from build123d import *

# Parameters (mm, degrees)
DODANIE_WYCI_GNI_CIE1_DEPTH = 5
SZKIC1_R                    = 3.5
WYTNIJ_WYCI_GNI_CIE1_DEPTH  = 88.4
SZKIC3_R                    = 1.5
WYTNIJ_WYCI_GNI_CIE3_DEPTH  = 5
SZKIC5_R                    = 3
WYTNIJ_WYCI_GNI_CIE4_DEPTH  = 2.4
DODANIE_WYCI_GNI_CIE2_START = 5
DODANIE_WYCI_GNI_CIE2_DEPTH = 5
SZKIC7_R                    = 3.5
WYTNIJ_WYCI_GNI_CIE5_DEPTH  = 5
SZKIC8_R                    = 3.5
WYTNIJ_WYCI_GNI_CIE6_DEPTH  = 5
SZKIC9_R                    = 1.5
WYTNIJ_WYCI_GNI_CIE7_DEPTH  = 3
SZKIC10_R                   = 2.85
WYTNIJ_WYCI_GNI_CIE8_DEPTH  = 2
SZKIC11_W                   = 7
SZKIC11_H                   = 5
WYTNIJ_WYCI_GNI_CIE9_DEPTH  = 3.5


with BuildPart() as part:
    # outer-wire → Dodanie-wyciągnięcie1 (new body)
    with BuildSketch(Plane.XY):
        with BuildLine():
            Line((-24, -24.53020641), (62.5, -24.53020641))
            ThreePointArc((62.5, -24.53020641), (65.803504247, -23.968789974), (68.736080178, -22.347578348))
            Line((68.736080178, -22.347578348), (89, -6.182628062))
            ThreePointArc((89, -6.182628062), (91.932575931, -4.561416436), (95.236080178, -4))
            Line((95.236080178, -4), (167, -4))
            ThreePointArc((167, -4), (172.310885546, -5.526836794), (176, -9.641101056))
            Line((176, -9.641101056), (192, -39.280484771))
            ThreePointArc((192, -39.280484771), (195.676368139, -43.118069462), (200.799707694, -44.53020641))
            Line((200.799707694, -44.53020641), (271, -44.53020641))
            ThreePointArc((271, -44.53020641), (292.697243682, -34.454979346), (299, -11.3778078))
            Line((299, -11.3778078), (299, 70.236479581))
            ThreePointArc((299, 70.236479581), (290.082226047, 86.530998263), (273, 93.827270232))
            Line((273, 93.827270232), (-19, 110))
            ThreePointArc((-19, 110), (-33.142135624, 104.142135624), (-39, 90))
            Line((-39, 90), (-39, -9.53020641))
            ThreePointArc((-39, -9.53020641), (-34.606601718, -20.136808128), (-24, -24.53020641))
        make_face()
    extrude(amount=DODANIE_WYCI_GNI_CIE1_DEPTH)

    # Szkic1 → Wytnij-wyciągnięcie1 (cut)
    with BuildSketch(Plane(origin=(0, -24.53020641, 0), x_dir=(-1, 0, 0), z_dir=(0, -1, 0))):
        with Locations((19, 0)):
            Circle(SZKIC1_R)
    extrude(amount=-WYTNIJ_WYCI_GNI_CIE1_DEPTH, mode=Mode.SUBTRACT)

    # Szkic3 → Wytnij-wyciągnięcie3 (cut)
    with BuildSketch(Plane.XY.offset(5)):
        with Locations((-5, 77.5)):
            Circle(SZKIC3_R)
        with Locations((-29, 77.5)):
            Circle(SZKIC3_R)
        with Locations((-29, -12.5)):
            Circle(SZKIC3_R)
        with Locations((-29, 32.5)):
            Circle(SZKIC3_R)
        with Locations((-5, 32.5)):
            Circle(SZKIC3_R)
        with Locations((-5, -12.5)):
            Circle(SZKIC3_R)
    extrude(amount=-WYTNIJ_WYCI_GNI_CIE3_DEPTH, mode=Mode.SUBTRACT)

    # Szkic5 → Wytnij-wyciągnięcie4 (cut)
    with BuildSketch(Plane.XY.offset(5)):
        with Locations((-29, -12.5)):
            Circle(SZKIC5_R)
        with Locations((-29, 32.5)):
            Circle(SZKIC5_R)
        with Locations((-29, 77.5)):
            Circle(SZKIC5_R)
        with Locations((-5, 77.5)):
            Circle(SZKIC5_R)
        with Locations((-5, 32.5)):
            Circle(SZKIC5_R)
        with Locations((-5, -12.5)):
            Circle(SZKIC5_R)
    extrude(amount=-WYTNIJ_WYCI_GNI_CIE4_DEPTH, mode=Mode.SUBTRACT)

    # Szkic6 → Dodanie-wyciągnięcie2 (add)
    with BuildSketch(Plane(origin=(0, 0, 0), x_dir=(-1, 0, 0), z_dir=(0, 0, -1)).offset(DODANIE_WYCI_GNI_CIE2_START)):
        with BuildLine():
            Line((-8, -24.53020641), (-8, 108.504576357))
            Line((-8, 108.504576357), (-273, 93.827270232))
            ThreePointArc((-273, 93.827270232), (-290.082226047, 86.530998263), (-299, 70.236479581))
            Line((-299, 70.236479581), (-299, -11.3778078))
            ThreePointArc((-299, -11.3778078), (-292.697243682, -34.454979346), (-271, -44.53020641))
            Line((-271, -44.53020641), (-200.799707694, -44.53020641))
            ThreePointArc((-200.799707694, -44.53020641), (-195.676368139, -43.118069462), (-192, -39.280484771))
            Line((-192, -39.280484771), (-176, -9.641101056))
            ThreePointArc((-176, -9.641101056), (-172.310885546, -5.526836794), (-167, -4))
            Line((-167, -4), (-95.236080178, -4))
            ThreePointArc((-95.236080178, -4), (-91.932575931, -4.561416436), (-89, -6.182628062))
            Line((-89, -6.182628062), (-68.736080178, -22.347578348))
            ThreePointArc((-68.736080178, -22.347578348), (-65.803504247, -23.968789974), (-62.5, -24.53020641))
            Line((-62.5, -24.53020641), (-8, -24.53020641))
        make_face()
    extrude(amount=-DODANIE_WYCI_GNI_CIE2_DEPTH)

    # Szkic7 → Wytnij-wyciągnięcie5 (cut)
    with BuildSketch(Plane(origin=(0, 65.36979359, 0), x_dir=(-1, 0, 0), z_dir=(0, -1, 0))):
        with Locations((19, 0)):
            Circle(SZKIC7_R)
    extrude(amount=-WYTNIJ_WYCI_GNI_CIE5_DEPTH, mode=Mode.SUBTRACT)

    # Szkic8 → Wytnij-wyciągnięcie6 (cut)
    with BuildSketch(Plane(origin=(0, 73.36979359, 0), x_dir=(-1, 0, 0), z_dir=(0, -1, 0))):
        with Locations((19, 0)):
            Circle(SZKIC8_R)
    extrude(amount=-WYTNIJ_WYCI_GNI_CIE6_DEPTH, mode=Mode.SUBTRACT)

    # Szkic9 → Wytnij-wyciągnięcie7 (cut)
    with BuildSketch(Plane(origin=(0, 73.36979359, 0), x_dir=(-1, 0, 0), z_dir=(0, -1, 0))):
        with Locations((19, 0)):
            Circle(SZKIC9_R)
    extrude(amount=WYTNIJ_WYCI_GNI_CIE7_DEPTH, mode=Mode.SUBTRACT)

    # Szkic10 → Wytnij-wyciągnięcie8 (cut)
    with BuildSketch(Plane(origin=(0, 65.36979359, 0), x_dir=(-1, 0, 0), z_dir=(0, -1, 0))):
        with Locations((19, 0)):
            Circle(SZKIC10_R)
    extrude(amount=WYTNIJ_WYCI_GNI_CIE8_DEPTH, mode=Mode.SUBTRACT)

    # Szkic11 → Wytnij-wyciągnięcie9 (cut)
    with BuildSketch(Plane(origin=(0, 0, 0), x_dir=(-1, 0, 0), z_dir=(0, 0, -1))):
        with Locations((19, 75.86979359)):
            Rectangle(SZKIC11_W, SZKIC11_H)
        with Locations((19, 67.86979359)):
            Rectangle(SZKIC11_W, SZKIC11_H)
    extrude(amount=-WYTNIJ_WYCI_GNI_CIE9_DEPTH, mode=Mode.SUBTRACT)


solid = part.part
Work out the finished part from the listing and answer in its coordinate system (mm). A direction names the side the tool comes from. Give positions to 0.01 mm unless a question says otherwise; leave off trailing zeros. Loops run counter-clockwise (first coordinate to the right, second up) from the corner with the lowest first, then second, coordinate; pieces in that order, holes last. Notation, with made-up numbers: (-11, -24.5) - (47, -24.5) arc R27 cw to (47, 1.5) - close; hole circle Ø10 at (-22, 20). An arc over 180 degrees is marked (long way). Answer in a Markdown table with one row per item. Add a question column.
Q1. The part is cut by section C-C (x = 120). Determine the outline of the cut face in (y, z), and give its area (3 significant figures).
Q2. Each of these flat-tipped pins is pushed along its axis until it touches: P1, Ø5.5, axis at x = -29, y = 32.5, coming from the +Z side; P2, Ø8, axis at x = -29, y = -12.5, coming from the -Z side; P3, Ø1.5, axis at x = 205.5, z = 0.5, coming from the +Y side. Where does it stop, or does it pass through?
Q3. Determine the mould class of faces 1 (the flat face through (156, 33, -5)), 2 (the flat face through (-4, -11, 2.6)), 3 (the flat face through (29, -24.53, 0)) for opening direction Y: released by +Y, released by -Y, zero draft, split by the parting line, or undercut.
Q4. A tool of negligible diameter and unlimited length cuts with its end or side. For faces 4 (the flat face through (299, 30, 0)), 5 (the flat face through (128, 34, 5)), 6 (the cylindrical face through (91.977, -4.546, -0.07)), 7 (the flat face through (-28, 79, 2.6)), from which of +Z, -Z, +X, -X, +Y, -Y can it reach the whole face along a straight path? Write none if from no direction.
Q5. Consider line 1 along Y through (x, z) = (-5, 1.6); line 2 along X through (y, z) = (77.5, 1.55); line 3 along Y through (x, z) = (-29, 1.5). Determine where each line is inside the solid, lowest interval first.
Q6. The part is cut by section B-B (y = -28.5). Determine the outline of the cut face in (x, z), and give its area (3 significant figures).
Q7. The part is cut by section A-A (z = -2). Determine the outline of the cut face in (x, y).
Solution:
| question | item | result |
|---|---|---|
| 1 | outline | (-4, -5) - (102.3, -5) - (102.3, 5) - (-4, 5) - close |
| 1 | area | 1,060 mm² |
| 2 | P1 | stops at z = 2.6 |
| 2 | P2 | stops at z = 0 |
| 2 | P3 | stops at y = 97.61 |
| 3 | face 1 | zero draft |
| 3 | face 2 | undercut |
| 3 | face 3 | released by -Y |
| 4 | face 4 | +Z, -Z, +X, +Y |
| 4 | face 5 | +Z, +X, -X, +Y, -Y |
| 4 | face 6 | +Z, -Z, -Y |
| 4 | face 7 | +Z |
| 5 | line 1 | y = -24.53 to -14, -11 to 31, 34 to 76, 79 to 109.22 |
| 5 | line 2 | x = -39 to -30.5, -27.5 to -22.5, -15.5 to -6.5, -3.5 to 296.74 |
| 5 | line 3 | y = -23.67 to -14, -11 to 31, 34 to 76, 79 to 107.32 |
| 6 | outline | (186.18, -5) - (296.56, -5) - (296.56, 5) - (186.18, 5) - close |
| 6 | area | 1,100 mm² |
| 7 | outline | (8, -24.53) - (62.5, -24.53) arc R10 ccw to (68.74, -22.35) - (89, -6.18) arc R10 cw to (95.24, -4) - (167, -4) arc R10 cw to (176, -9.64) - (192, -39.28) arc R10 ccw to (200.8, -44.53) - (271, -44.53) arc R28.4 ccw to (299, -11.38) - (299, 70.24) arc R28.4 ccw to (273, 93.83) - (8, 108.5) - close |
